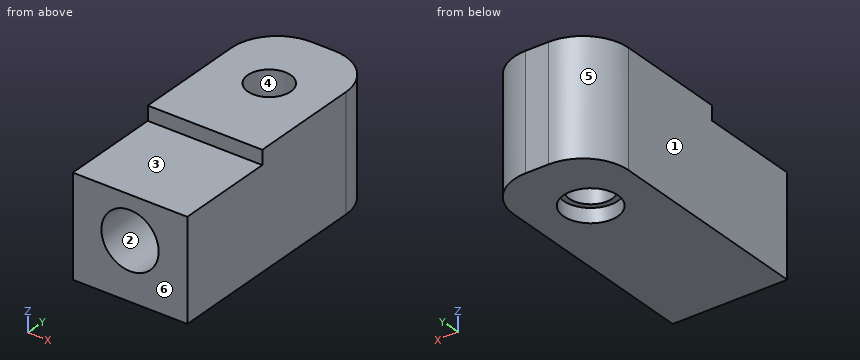
```python
from build123d import *

# Parameters (mm, degrees)
SKETCH2_W           = 10
SKETCH2_H           = 8.75
BOSS_EXTRUDE1_DEPTH = 8.75
SKETCH3_W           = 10
SKETCH3_H           = 10
BOSS_EXTRUDE2_DEPTH = 13.75
FILLET1_R           = 4
SKETCH4_R           = 2.5
CUT_EXTRUDE1_DEPTH  = 11.88
SKETCH5_R           = 1.875
CUT_EXTRUDE2_DEPTH  = 8.75
SKETCH6_R           = 2.375
CUT_EXTRUDE3_DEPTH  = 1.25


with BuildPart() as part:
    # Sketch2 → Boss-Extrude1 (new body)
    with BuildSketch(Plane.XY):
        with Locations((0, -6.875)):
            Rectangle(SKETCH2_W, SKETCH2_H)
    extrude(amount=BOSS_EXTRUDE1_DEPTH)

    # Sketch3 → Boss-Extrude2 (add)
    with BuildSketch(Plane(origin=(0, -2.5, 0), x_dir=(1, 0, 0), z_dir=(0, 1, 0))):
        with Locations((0, -5)):
            Rectangle(SKETCH3_W, SKETCH3_H)
    extrude(amount=BOSS_EXTRUDE2_DEPTH)

    # Fillet1
    fillet1_edges = [part.edges().sort_by_distance(p)[0] for p in [
        (5, 11.25, 5),
        (-5, 11.25, 5),
    ]]
    fillet(fillet1_edges, radius=FILLET1_R)

    # Sketch4 → Cut-Extrude1 (cut)
    with BuildSketch(Plane.XZ.offset(11.25)):
        with Locations((0, 5)):
            Circle(SKETCH4_R)
    extrude(amount=-CUT_EXTRUDE1_DEPTH, mode=Mode.SUBTRACT)

    # Sketch5 → Cut-Extrude2 (cut)
    with BuildSketch(Plane.XY.offset(10)):
        with Locations((0, 5)):
            Circle(SKETCH5_R)
    extrude(amount=-CUT_EXTRUDE2_DEPTH, mode=Mode.SUBTRACT)

    # Sketch6 → Cut-Extrude3 (cut)
    with BuildSketch(Plane(origin=(0, 0, 0), x_dir=(-1, 0, 0), z_dir=(0, 0, -1))):
        with Locations((0, 5)):
            Circle(SKETCH6_R)
    extrude(amount=-CUT_EXTRUDE3_DEPTH, mode=Mode.SUBTRACT)


solid = part.part
```
Model file for the job. Use its own axes, mm. Face numbers are marked on the shaded views. A direction names the side the tool comes from. Give positions to 0.01 mm unless a question says otherwise; leave off trailing zeros. Write each loop counter-clockwise with the first axis right and the second up, starting at its lowest first coordinate (ties: lowest second). Pieces come first, ordered by that corner, then holes. Notation, with made-up numbers: M -2,-15 L 47,-15 A16 ccw 47,-10 Z; hole C -8.75,28 d11. An arc over 180 degrees is marked long. Use a Markdown table: item, result.
1) Cut at A-A (x = 0). List the corners of the cut face in (y, z) (3 decimals), and give its area (3 significant figures).
Responses:
| item | result |
|---|---|
| outline | M -11.25,0 L 2.625,0 L 2.625,1.25 L 3.125,1.25 L 3.125,10 L -2.5,10 L -2.5,8.75 L -11.25,8.75 L -11.25,7.5 L 0.63,7.5 L 0.63,2.5 L -11.25,2.5 Z; M 6.875,1.25 L 7.375,1.25 L 7.375,0 L 11.25,0 L 11.25,10 L 6.875,10 Z |
| area | 116 mm2 |
2) Pull direction Y, two halves, no side cores. Call the marked faces 3, 4, 5 and 6: +Y half, -Y half, draft (parallel to the pull), parting line (faces both ways), or undercut.
Responses:
| item | result |
|---|---|
| face 3 | draft |
| face 4 | undercut |
| face 5 | +Y half |
| face 6 | -Y half |
3) Cut at C-C (y = 5). List the corners of the cut face in (x, z) (3 decimals).
Responses:
| item | result |
|---|---|
| outline | M -5,0 L -2.375,0 L -2.375,1.25 L -1.875,1.25 L -1.875,10 L -5,10 Z; M 1.875,1.25 L 2.375,1.25 L 2.375,0 L 5,0 L 5,10 L 1.875,10 Z |
4) Drill centre lines: line 1 (Y direction, x = 0, z = 0.8) (3 decimals); line 2 (Z direction, x = 0, y = -6.5); line 3 (Y direction, x = 0, z = 6) (3 decimals). Where is each one in solid material? Low to high. Write a range as from..to.
Responses:
| item | result |
|---|---|
| line 1 | y = -11.25..2.625, 7.375..11.25 |
| line 2 | z = 0..2.5, 7.5..8.75 |
| line 3 | y = 0.63..3.125, 6.875..11.25 |
5) Cut at D-D (y = -0.75). List the corners of the cut face in (x, z).
Responses:
| item | result |
|---|---|
| outline | M -5,0 L 5,0 L 5,10 L -5,10 Z; hole C 0,5 d5 |
6) Cut at B-B (z = 5). List the corners of the cut face in (x, y) (3 decimals), and give its area (3 significant figures).
Responses:
| item | result |
|---|---|
| outline | M -5,-11.25 L -2.5,-11.25 L -2.5,0.63 L 2.5,0.63 L 2.5,-11.25 L 5,-11.25 L 5,7.25 A4 ccw 1,11.25 L -1,11.25 A4 ccw -5,7.25 Z; hole C 0,5 d3.75 |
| area | 148 mm2 |
7) Tool access for the marked faces 1 and 2: list every direction of +Z, -Z, +X, -X, +Y, -Y with a clear straight run to the whole face (end or side of a thin tool).
Responses:
| item | result |
|---|---|
| face 1 | +Z, -Z, -X, +Y, -Y |
| face 2 | -Y |
8) Pin check, flat tips, straight feed: pin 1 (5 mm diameter, centred on x = 0, y = 5, fed in from +Z); pin 2 (1.5 mm diameter, centred on x = 0, z = 4, fed in from -Y); pin 3 (1.4 mm diameter, centred on x = -1, y = 4.5, fed in from -Z). Stop position of each tip, or through.
Responses:
| item | result |
|---|---|
| pin 1 | stops at z = 10 |
| pin 2 | stops at y = 0.63 |
| pin 3 | passes through |
